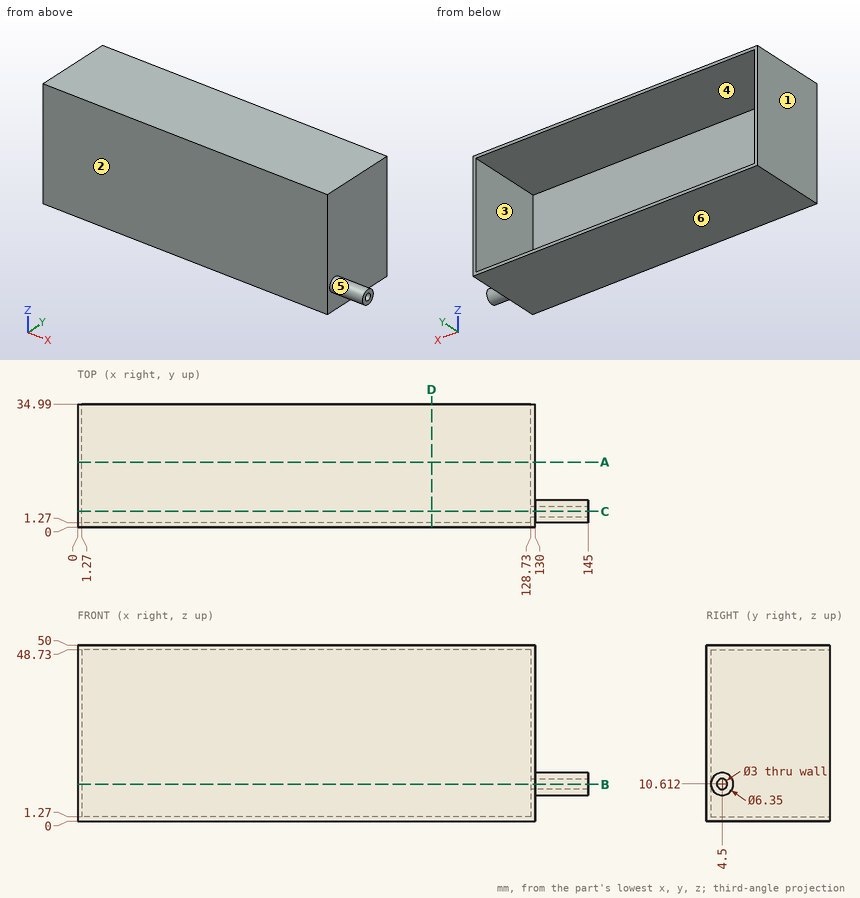
Part print with two shaded views. Sizes in mm from the minimum x, y, z corner. A direction names the side the tool comes from. Give positions to 0.01 mm unless a question says otherwise; leave off trailing zeros. Order: outer loops, then holes, each group sorted by start corner. A loop starts at its lowest first (then second) coordinate and runs counter-clockwise, first axis right, second up.
1) Saw through at B-B, the plane z = 10.5. Write the cut outline in (x, y), then the cut area to 3 significant figures.
2) Saw through at A-A, the plane y = 18.5. Write the cut outline in (x, z).
3) Saw through at C-C, the plane y = 4.5. Write the cut outline in (x, z).
4) Saw through at D-D, the plane x = 100.5. Write the cut outline in (y, z), then the cut area to 3 significant figures.
5) 3-axis set-ups, long thin cutter, end or side, ignore diameter. For the marked faces 4, 5 and 6: which of +Z, -Z, +X, -X, +Y, -Y reach the whole face in a straight line?
6) Mould opens along X. For the marked faces 1, 2 and 3 say: +X half, -X half, draft (parallel to the pull), parting line (faces both ways), or undercut.
7) Pin check, flat tips, straight feed: pin 1 (2 mm diameter, centred on x = 64, z = 21.5, fed in from +Y); pin 2 (10 mm diameter, centred on y = 18, z = 35, fed in from +X). Stop position of each tip, or through.
8) Wall check: probe 1 along Z at (x, y) = (104, 24); probe 2 along X at (y, z) = (14.5, 43); probe 3 along Y at (x, z) = (54, 37). Give the ranges that are in metal, low to high.
Computed:
1. outline: (0, 0) - (130, 0) - (130, 1.33) - (145, 1.33) - (145, 3) - (128.73, 3) - (128.73, 1.27) - (1.27, 1.27) - (1.27, 34.99) - (0, 34.99) - close; (128.73, 6) - (145, 6) - (145, 7.67) - (130, 7.67) - (130, 34.99) - (128.73, 34.99) - close
1. area: 297 mm2
2. outline: (0, 0) - (130, 0) - (130, 50) - (0, 50) - close; hole (1.27, 1.27) - (128.73, 1.27) - (128.73, 48.73) - (1.27, 48.73) - close
3. outline: (0, 0) - (130, 0) - (130, 7.44) - (145, 7.44) - (145, 9.11) - (128.73, 9.11) - (128.73, 1.27) - (1.27, 1.27) - (1.27, 48.73) - (128.73, 48.73) - (128.73, 12.11) - (145, 12.11) - (145, 13.79) - (130, 13.79) - (130, 50) - (0, 50) - close
4. outline: (0, 0) - (34.99, 0) - (34.99, 1.27) - (1.27, 1.27) - (1.27, 48.73) - (34.99, 48.73) - (34.99, 50) - (0, 50) - close
4. area: 149 mm2
5. face 4: +Y
5. face 5: +X
5. face 6: -Z, +X, -X, +Y, -Y
6. face 1: -X half
6. face 2: draft
6. face 3: undercut
7. pin 1: stops at y = 1.27
7. pin 2: stops at x = 130
8. probe 1: z = 0 to 1.27, 48.73 to 50
8. probe 2: x = 0 to 1.27, 128.73 to 130
8. probe 3: y = 0 to 1.27
